Input: part model. Units: mm. Frame: model coordinates. A direction names the side the tool comes from. Coordinates: 2 decimals unless noted, no trailing zeros. Order: outer loops, then holes, each group sorted by start corner. A loop starts at its lowest first (then second) coordinate and runs counter-clockwise, first axis right, second up. Notation, with made-up numbers: (-38.5, 4.5) -> (-30.5, 4.5) arc R23 cw to (-30.5, 30.5) -> close; hole circle Ø10 at (76.25, 62). An arc over 180 degrees is marked (long way). Write each question's results on one line, items separated by ' | '.
```python
from build123d import *

# Parameters (mm, degrees)
SKETCH1_R           = 34
BOSS_EXTRUDE1_DEPTH = 101
SKETCH2_R           = 4
BOSS_EXTRUDE2_DEPTH = 27.5
SKETCH3_R           = 2.225
CUT_EXTRUDE1_DEPTH  = 20
SKETCH4_R           = 14
BOSS_EXTRUDE3_DEPTH = 7


with BuildPart() as part:
    # Sketch1 → Boss-Extrude1 (new body)
    with BuildSketch(Plane.XY):
        Circle(SKETCH1_R)
    extrude(amount=BOSS_EXTRUDE1_DEPTH)

    # Sketch2 → Boss-Extrude2 (add)
    with BuildSketch(Plane.XY.offset(101)):
        Circle(SKETCH2_R)
    extrude(amount=BOSS_EXTRUDE2_DEPTH)

    # Sketch3 → Cut-Extrude1 (cut)
    with BuildSketch(Plane.XY.offset(101)):
        with Locations((-18.375, 10.608811196)):
            Circle(SKETCH3_R)
        with Locations((18.375, 10.608811196)):
            Circle(SKETCH3_R)
        with Locations((0, -21.217622393)):
            Circle(SKETCH3_R)
    extrude(amount=-CUT_EXTRUDE1_DEPTH, mode=Mode.SUBTRACT)

    # Sketch4 → Boss-Extrude3 (add)
    with BuildSketch(Plane(origin=(0, 0, 0), x_dir=(-1, 0, 0), z_dir=(0, 0, -1))):
        Circle(SKETCH4_R)
    extrude(amount=BOSS_EXTRUDE3_DEPTH)


solid = part.part
```
(1) Cut plane D-D, the plane y = 19. Return loops of the section in (x, z), plus the area to 3 significant figures.
Return value:
outline: (-28.2, 0) -> (28.2, 0) -> (28.2, 101) -> (-28.2, 101) -> close | area: 5,700 mm2
(2) Cut plane C-C, the plane z = 109. Return loops of the section in (x, y).
Return value:
outline: circle Ø8 at (0, 0)
(3) Mould query, pull axis Y, two halves, no side actions, for faces 4 (the face through (-12.932, -5.362, -3.451)), 5 (the face through (18, 11, 81)), 6 (the face through (7, 0, 101)). Classes: +Y half, -Y half, draft (parallel to the pull), parting line (faces both ways), or undercut.
Return value:
face 4: parting line | face 5: undercut | face 6: draft
(4) Pin query (flat end, axial travel): P1, Ø10, axis at y = -20.5, z = 72, coming from the -X side; P2, Ø1.3, axis at x = -19, y = 9.5, coming from the +Z side; P3, Ø3.5, axis at x = 0.5, y = -20, coming from the +Z side. Return the tip coordinate at first contact, or that it passes through.
Return value:
P1: x = -30.26 | P2: z = 81 | P3: z = 101
(5) Line query: line 1 along Z through (x, y) = (-24, -8.5); line 2 along Z through (x, y) = (6, -11); line 3 along Y through (x, z) = (-18.5, 84). Output: solid intervals per line, ascending. Write a range as from..to.
Return value:
line 1: 0..101 | line 2: -7..101 | line 3: -28.53..8.39, 12.83..28.53
(6) Reachability of faces 1 (the face through (-18, 11, 81)), 2 (the face through (15, 0, 0)), 3 (the face through (0, 0, -7)) from +Z, -Z, +X, -X, +Y, -Y: full face, straight path, thin tool, end or side. Return the list, or none.
Return value:
face 1: +Z | face 2: -Z | face 3: -Z, +X, -X, +Y, -Y
(7) Cut plane B-B, the plane x = 0. Return loops of the section in (y, z).
Return value:
outline: (-34, 0) -> (-14, 0) -> (-14, -7) -> (14, -7) -> (14, 0) -> (34, 0) -> (34, 101) -> (4, 101) -> (4, 128.5) -> (-4, 128.5) -> (-4, 101) -> (-18.99, 101) -> (-18.99, 81) -> (-23.44, 81) -> (-23.44, 101) -> (-34, 101) -> close
(8) Cut plane A-A, the plane y = 0. Return loops of the section in (x, z).
Return value:
outline: (-34, 0) -> (-14, 0) -> (-14, -7) -> (14, -7) -> (14, 0) -> (34, 0) -> (34, 101) -> (4, 101) -> (4, 128.5) -> (-4, 128.5) -> (-4, 101) -> (-34, 101) -> close
